Answer from the drawing. Dimensions are ordinates in mm from the lowest x, y and z of the part. A direction names the side the tool comes from. Coordinates: 2 decimals unless noted, no trailing zeros. Order: outer loops, then holes, each group sorted by start corner. A loop starts at its lowest first (then second) coordinate and runs counter-clockwise, first axis right, second up. Notation, with made-up numbers: M -33,-34 L 22,-34 A29 cw 22,-10 Z; hole C 17,-27 d11. An arc over 180 degrees is marked long. Use a Markdown table: item, result.
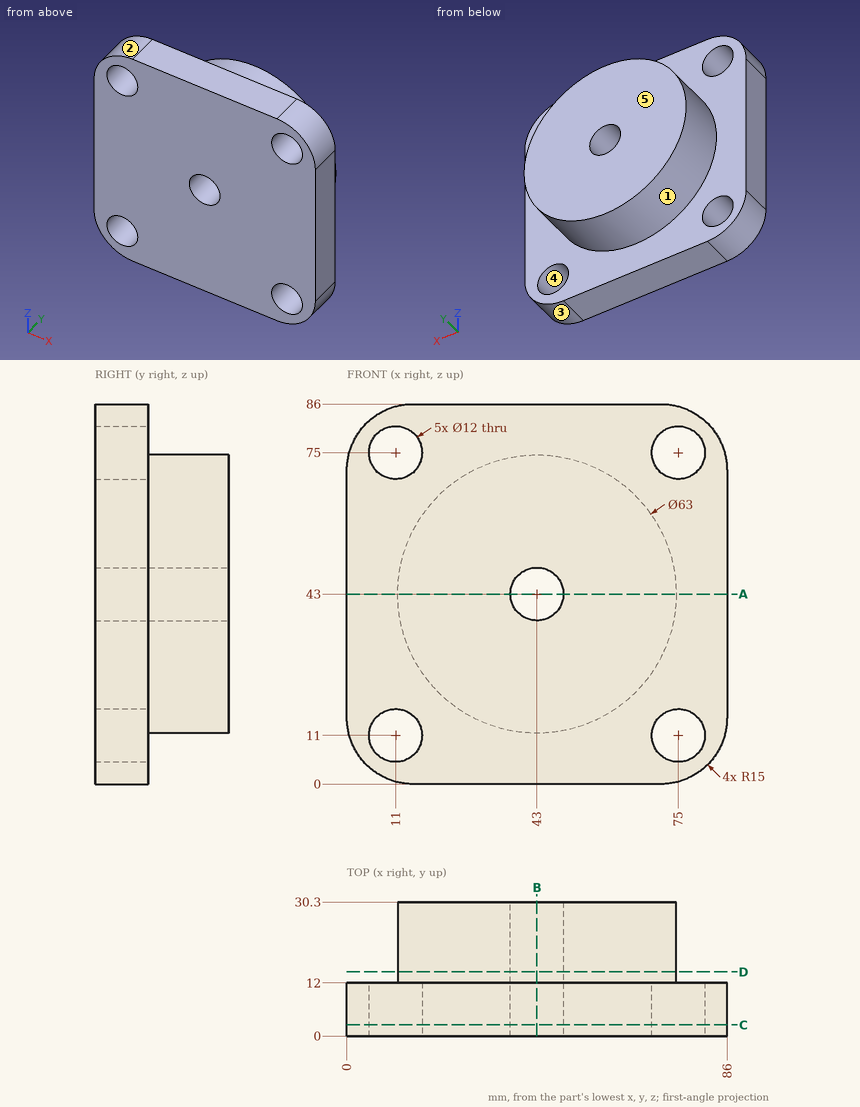
(1) Given P1, Ø10, axis at x = 57, y = 26.5, coming from the -Z side; P2, Ø9.5, axis at x = 75, z = 75, coming from the +Y side; P3, Ø2, axis at x = 74.5, z = 58, coming from the +Y side; P4, Ø1, axis at y = 20.5, z = 67.5, coming from the +X side, each flat-ended and moving along its own axis, determine where each tip first touches the part or whether it passes through.
Conclusion:
| item | result |
|---|---|
| P1 | z = 12.81 |
| P2 | through |
| P3 | y = 12 |
| P4 | x = 63.4 |
(2) A cutting plane is placed at D-D (y = 14.5). Determine the outline of the cut face in (x, z), then the cut area to 3 significant figures.
Conclusion:
| item | result |
|---|---|
| outline | C 43,43 d63; hole C 43,43 d12 |
| area | 3,000 mm2 |
(3) Straight lines are drawn through the part: L1, parallel to Z at x = 43, y = 22; L2, parallel to X at y = 9, z = 75; L3, parallel to Y at x = 35, z = 12.5. For each, find the intervals that lie inside material, in ascending order.
Conclusion:
| item | result |
|---|---|
| L1 | 11.5 to 37, 49 to 74.5 |
| L2 | 0.54 to 5, 17 to 69, 81 to 85.46 |
| L3 | 0 to 12 |
(4) A cutting plane is placed at B-B (x = 43). Determine the outline of the cut face in (y, z), then the cut area to 3 significant figures.
Conclusion:
| item | result |
|---|---|
| outline | M 0,0 L 12,0 L 12,11.5 L 30.3,11.5 L 30.3,37 L 0,37 Z; M 0,49 L 30.3,49 L 30.3,74.5 L 12,74.5 L 12,86 L 0,86 Z |
| area | 1,820 mm2 |
(5) Which of the six approach directions +Z, -Z, +X, -X, +Y, -Y give full straight-line access (tool end or side, diameter ignored) to the marked faces 1 and 2?
Conclusion:
| item | result |
|---|---|
| face 1 | +Y |
| face 2 | +Z, -X, +Y, -Y |
(6) A cutting plane is placed at A-A (z = 43). Determine the outline of the cut face in (x, y), then the cut area to 3 significant figures.
Conclusion:
| item | result |
|---|---|
| outline | M 0,0 L 37,0 L 37,30.3 L 11.5,30.3 L 11.5,12 L 0,12 Z; M 49,0 L 86,0 L 86,12 L 74.5,12 L 74.5,30.3 L 49,30.3 Z |
| area | 1,820 mm2 |
(7) A cutting plane is placed at C-C (y = 2.5). Determine the outline of the cut face in (x, z).
Conclusion:
| item | result |
|---|---|
| outline | M 0,15 A15 ccw 15,0 L 71,0 A15 ccw 86,15 L 86,71 A15 ccw 71,86 L 15,86 A15 ccw 0,71 Z; hole C 11,11 d12; hole C 11,75 d12; hole C 43,43 d12; hole C 75,11 d12; hole C 75,75 d12 |
(8) Determine the mould class of the marked faces 3, 4 and 5 for opening direction Z: pulls with the +Z half, pulls with the -Z half, needs draft (parallel to the pull), parting line crosses it, or undercut.
Conclusion:
| item | result |
|---|---|
| face 3 | pulls with the -Z half |
| face 4 | undercut |
| face 5 | needs draft |
